Check sheet for the drawn part. Datum: minimum x, y, z corner. Units: mm. A direction names the side the tool comes from. Coordinates: 2 decimals unless noted, no trailing zeros. Write each loop counter-clockwise with the first axis right and the second up, starting at its lowest first coordinate (ties: lowest second). Pieces come first, ordered by that corner, then holes. Notation, with made-up numbers: M -18.5,43 L 12.5,43 A13 ccw 12.5,56 Z; hole C 18,-14 d4. An arc over 180 degrees is marked long. Answer as a JSON object with one key per item and string values. Group by question number.
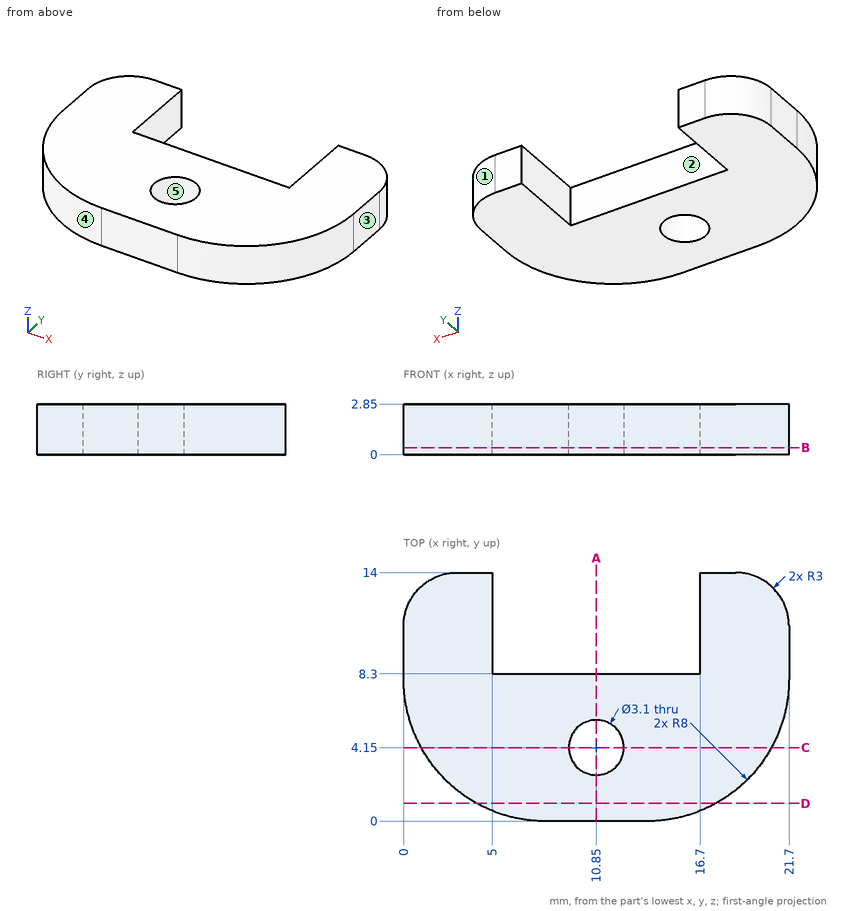
1) Set-up check for the marked faces 1 and 2: record each of +Z, -Z, +X, -X, +Y, -Y from which the full face is reachable in a straight line by a thin tool's end or side.
2) Section check D-D (y = 1). Record the cut outline in (x, z), then the cut area to 3 significant figures.
3) Go/stop test with flat-tipped pins: pin 1 Ø1 at (x, z) = (8, 1.5) entering from +Y; pin 2 Ø1.5 at (x, z) = (5, 1.5) entering from -Y; pin 3 Ø0.9 at (y, z) = (12, 1.5) entering from +X. Record where each tip stops, or that it passes through.
4) Section check B-B (z = 0.4). Record the cut outline in (x, y), then the cut area to 3 significant figures.
5) Section check C-C (y = 4.15). Record the cut outline in (x, z), then the cut area to 3 significant figures.
6) Material ranges on probe 1 along Y at (x, z) = (10.85, 0.6); probe 2 along Y at (x, z) = (12.5, 0.4); probe 3 along X at (y, z) = (5.5, 1.2), recorded low to high. Write a range as [from, to].
7) Draft check along Y on the marked faces 3, 4 and 5. Enter one of: +Y half, -Y half, draft (parallel to the pull), parting line (faces both ways), or undercut.
8) Section check A-A (x = 10.85). Record the cut outline in (y, z).
Entries:
{
 "1": {"face 1": "+Z, -Z, +X, +Y", "face 2": "+Z, -Z, +Y"},
 "2": {"outline": "M 4.13,0 L 17.57,0 L 17.57,2.85 L 4.13,2.85 Z", "area": "38.3 mm^2"},
 "3": {"pin 1": "y = 8.3", "pin 2": "y = 0.32", "pin 3": "x = 21.65"},
 "4": {"outline": "M 0,8 A8 ccw 8,0 L 13.7,0 A8 ccw 21.7,8 L 21.7,11 A3 ccw 18.7,14 L 16.7,14 L 16.7,8.3 L 5,8.3 L 5,14 L 3,14 A3 ccw 0,11 Z; hole C 10.85,4.15 d3.1", "area": "198 mm^2"},
 "5": {"outline": "M 0.99,0 L 9.3,0 L 9.3,2.85 L 0.99,2.85 Z; M 12.4,0 L 20.71,0 L 20.71,2.85 L 12.4,2.85 Z", "area": "47.4 mm^2"},
 "6": {"probe 1": "[0, 2.6], [5.7, 8.3]", "probe 2": "[0, 8.3]", "probe 3": "[0.4, 10.09], [11.61, 21.3]"},
 "7": {"face 3": "draft", "face 4": "-Y half", "face 5": "undercut"},
 "8": {"outline": "M 0,0 L 2.6,0 L 2.6,2.85 L 0,2.85 Z; M 5.7,0 L 8.3,0 L 8.3,2.85 L 5.7,2.85 Z"}
}
